from build123d import *

# Parameters (mm, degrees)
F0_W     = 25.4
F0_H     = 50.8
F0_R     = 6.35
F1_DEPTH = 9.525
F2_SIZE  = 3.175
F4_D     = 16.66748
F4_DEPTH = 20.32
F4_TIP   = 5.0074161752


with BuildPart() as f1:
    # F0 (on Front) → F1 (new body, symmetric)
    with BuildSketch(Plane.XZ):
        Rectangle(F0_W, F0_H)
        with Locations((0, -12.7)):
            Circle(F0_R, mode=Mode.SUBTRACT)
    extrude(amount=F1_DEPTH, both=True)

    # F2
    f2_edges = [f1.edges().sort_by_distance(p)[0] for p in [
        (12.7, 0, -25.4),
        (-12.7, 0, -25.4),
    ]]
    chamfer(f2_edges, length=F2_SIZE)

    # F4
    with Locations(Plane.XY.offset(25.4)):
        with Locations((0, 0)):
            Hole(F4_D / 2, depth=F4_DEPTH)
            with Locations((0, 0, -(F4_DEPTH + F4_TIP / 2))):  # 118° drill point
                Cone(0, F4_D / 2, F4_TIP, mode=Mode.SUBTRACT)


solid = f1.part
Could you check a few things on this model? Use its own coordinates, in mm. Give positions to 0.01 mm unless a question says otherwise; leave off trailing zeros. Write each loop counter-clockwise with the first axis right and the second up, starting at its lowest first coordinate (ties: lowest second). Pieces come first, ordered by that corner, then holes. Notation, with made-up numbers: (-3.5, 32.5) -> (51.5, 32.5) arc R4 cw to (51.5, 36.5) -> close; hole circle Ø4 at (1, -38). An arc over 180 degrees is marked (long way). Answer as CSV lines item,"result". Start each with the question number.
(1) If we mould it in two halves opening along Y, with no side actions, what happens to faces 1 (the face through (8.326, 0.366, 15.098)), 2 (the face through (-1.38, 0.13, -18.9)), 3 (the face through (0, -9.525, 0)), 4 (the face through (0, 9.525, 0))? For each: +Y half, -Y half, draft (parallel to the pull), parting line (faces both ways), or undercut.
(2) I'm going to push flat-ended pins straight in: pin 1 Ø10 at (x, z) = (0, -12.7) entering from +Y; pin 2 Ø2 at (x, y) = (-4, 4) entering from +Z. Where does each tip first touch, or does it pass through?
(3) Please list where these lines run through material, in increasing order: line 1 (X direction, y = -4.5, z = -12.5); line 2 (X direction, y = 0, z = 14.5); line 3 (Y direction, x = 0, z = 17.25) (3 decimals).
(4) If we section it at B-B, the plane z = 15: Write out the boundary of the cut face in (x, y) (3 decimals).
(5) If we section it at A-A, the plane z = -12.7: Write out the boundary of the cut face in (x, y) (3 decimals).
Answer list:
1,face 1,"undercut"
1,face 2,"draft"
1,face 3,"-Y half"
1,face 4,"+Y half"
2,pin 1,"through"
2,pin 2,"z = 4.07"
3,line 1,"-12.7 to -6.35, 6.35 to 12.7"
3,line 2,"-12.7 to -8.33, 8.33 to 12.7"
3,line 3,"-9.525 to -8.334, 8.334 to 9.525"
4,outline,"(-12.7, -9.525) -> (12.7, -9.525) -> (12.7, 9.525) -> (-12.7, 9.525) -> close; hole circle Ø16.667 at (0, 0)"
5,outline,"(-12.7, -9.525) -> (-6.35, -9.525) -> (-6.35, 9.525) -> (-12.7, 9.525) -> close; (6.35, -9.525) -> (12.7, -9.525) -> (12.7, 9.525) -> (6.35, 9.525) -> close"
